from build123d import *

# Parameters (mm, degrees)
BOSS_EXTRUDE1_DEPTH     = 5
SKETCH2_W               = 3.5
SKETCH2_H               = 12
SKETCH2_W_2             = 3
BOSS_EXTRUDE2_DEPTH     = 20
SKETCH3_W               = 12
SKETCH3_H               = 3
SKETCH3_H_2             = 3.5
BOSS_EXTRUDE3_DEPTH     = 20
SKETCH4_W               = 5
SKETCH4_H               = 8
BOSS_EXTRUDE4_DEPTH     = 18
SKETCH5_R               = 3.5
CUT_EXTRUDE1_DEPTH      = 3.5
SKETCH6_R               = 3.5
CUT_EXTRUDE2_DEPTH      = 3.5
SKETCH7_R               = 1.625
CUT_EXTRUDE3_DEPTH      = 5
SKETCH8_R               = 2.5
CUT_EXTRUDE4_DEPTH      = 3
SKETCH9_R               = 2.5
CUT_EXTRUDE5_DEPTH      = 3
FILLET1_R               = 6
FILLET2_R               = 2
FILLET4_R               = 4
SURFACECUT2_START       = -20
SURFACECUT2_DEPTH       = 25
SURFACECUT2_START_2     = 5
SURFACECUT2_2_OUTLINE_W = 12
SURFACECUT2_2_OUTLINE_H = 3
SURFACECUT2_2_DEPTH     = 20


# Read off the part's stored shape, not the designer's step: SurfaceCut2
with BuildPart() as part:
    # Sketch1 → Boss-Extrude1 (new body)
    with BuildSketch(Plane.XY):
        Polygon((21.1, 0), (38.5, 0), (38.5, 12), (17.6, 12), (17.6, 26), (12.6, 26), (12.6, 12), (0, 12), (0, 0), (9.1, 0), (9.1, -26.5), (21.1, -26.5), align=None)
    extrude(amount=BOSS_EXTRUDE1_DEPTH)

    # Sketch2 → Boss-Extrude2 (add)
    with BuildSketch(Plane(origin=(0, 0, 0), x_dir=(-1, 0, 0), z_dir=(0, 0, -1))):
        with Locations((-1.75, 6)):
            Rectangle(SKETCH2_W, SKETCH2_H)
        with Locations((-37, 6)):
            Rectangle(SKETCH2_W_2, SKETCH2_H)
    extrude(amount=BOSS_EXTRUDE2_DEPTH)

    # Sketch3 → Boss-Extrude3 (add)
    with BuildSketch(Plane.XY.offset(5)):
        with Locations((15.1, -25)):
            Rectangle(SKETCH3_W, SKETCH3_H)
        with Locations((15.1, 10.25)):
            Rectangle(SKETCH3_W, SKETCH3_H_2)
    extrude(amount=BOSS_EXTRUDE3_DEPTH)

    # Sketch4 → Boss-Extrude4 (add)
    with BuildSketch(Plane(origin=(0, 0, 0), x_dir=(-1, 0, 0), z_dir=(0, 0, -1))):
        with Locations((-15.1, 22)):
            Rectangle(SKETCH4_W, SKETCH4_H)
    extrude(amount=BOSS_EXTRUDE4_DEPTH)

    # Sketch5 → Cut-Extrude1 (cut)
    with BuildSketch(Plane.ZY):
        with Locations((-14, 6)):
            Circle(SKETCH5_R)
    extrude(amount=-CUT_EXTRUDE1_DEPTH, mode=Mode.SUBTRACT)

    # Sketch6 → Cut-Extrude2 (cut)
    with BuildSketch(Plane(origin=(0, 12, 0), x_dir=(1, 0, 0), z_dir=(0, 1, 0))):
        with Locations(Location((15.1, -19, 0), (0, 0, 270))):
            Circle(SKETCH6_R)
    extrude(amount=-CUT_EXTRUDE2_DEPTH, mode=Mode.SUBTRACT)

    # Sketch7 → Cut-Extrude3 (cut)
    with BuildSketch(Plane.ZY.offset(-12.6)):
        with Locations((-14, 22)):
            Circle(SKETCH7_R)
    extrude(amount=-CUT_EXTRUDE3_DEPTH, mode=Mode.SUBTRACT)

    # Sketch8 → Cut-Extrude4 (cut)
    with BuildSketch(Plane.ZY.offset(-35.5)):
        with Locations((-14, 6)):
            Circle(SKETCH8_R)
    extrude(amount=-CUT_EXTRUDE4_DEPTH, mode=Mode.SUBTRACT)

    # Sketch9 → Cut-Extrude5 (cut)
    with BuildSketch(Plane(origin=(0, -23.5, 0), x_dir=(1, 0, 0), z_dir=(0, 1, 0))):
        with Locations(Location((15.1, -19, 0), (0, 0, 270))):
            Circle(SKETCH9_R)
    extrude(amount=-CUT_EXTRUDE5_DEPTH, mode=Mode.SUBTRACT)

    # Fillet1
    fillet1_edges = [part.edges().sort_by_distance(p)[0] for p in [
        (21.1, -25, 25),
        (9.1, -25, 25),
        (37, 0, -20),
        (37, 12, -20),
        (21.1, 10.25, 25),
        (9.1, 10.25, 25),
        (1.75, 0, -20),
        (1.75, 12, -20),
    ]]
    fillet(fillet1_edges, radius=FILLET1_R - 0.0001)  # a hair under: the kernel refuses the full size

    # Fillet2
    fillet2_edges = [part.edges().sort_by_distance(p)[0] for p in [
        (15.1, -26.5, 0),
        (38.5, 6, 5),
        (0, 6, 5),
        (15.1, 18, 0),
    ]]
    fillet(fillet2_edges, radius=FILLET2_R)

    # Fillet4
    fillet4_edges = [part.edges().sort_by_distance(p)[0] for p in [
        (15.1, 26, 5),
        (15.1, 26, -18),
        (15.1, 18, -18),
    ]]
    fillet(fillet4_edges, radius=FILLET4_R - 0.0001)  # a hair under: the kernel refuses the full size

    # SurfaceCut2 outline → SurfaceCut2 (cut)
    with BuildSketch(Plane.XY.offset(SURFACECUT2_START)):
        Polygon((0, 12), (0, 0), (9.1, 0), (9.1, -26.5), (21.1, -26.5), (21.1, 0), (38.5, 0), (38.5, 12), (17.6, 12), (17.6, 26), (12.6, 26), (12.6, 12), align=None)
    extrude(amount=SURFACECUT2_DEPTH, mode=Mode.SUBTRACT)

    # SurfaceCut2 2 outline → SurfaceCut2 2 (cut)
    with BuildSketch(Plane.XY.offset(SURFACECUT2_START_2)):
        with Locations((15.1, -25)):
            Rectangle(SURFACECUT2_2_OUTLINE_W, SURFACECUT2_2_OUTLINE_H)
    extrude(amount=SURFACECUT2_2_DEPTH, mode=Mode.SUBTRACT)


solid = part.part
Build history of the part. All positions in model axes, mm. Give positions to 0.01 mm unless a question says otherwise; leave off trailing zeros. Order: outer loops, then holes, each group sorted by start corner. A loop starts at its lowest first (then second) coordinate and runs counter-clockwise, first axis right, second up. Notation, with made-up numbers: M 49,6 L 54,6 A9 ccw 54,10 Z; hole C 79,-20.5 d4. An arc over 180 degrees is marked long. Put each result on its own line as item: value.
Item 1: Slice it at B-B, the plane x = 17.5. Write the cut outline in (y, z), plus the area to 3 significant figures.
From the geometry:
outline: M 8.5,5 L 12,5 L 12,16.45 L 8.5,16.45 Z; M 8.5,21.55 L 12,21.55 L 12,24.5 L 8.5,24.5 Z
area: 50.4 mm2
Item 2: Two-plate mould, pull along Z, no slides. Class faces 1 (the cylindrical face through (18.05, 10.27, 20.88)), 2 (the flat face through (15, 12, 13)), 3 (the flat face through (15, 10, 5)): +Z half, -Z half, draft (parallel to the pull), parting line (faces both ways), or undercut.
From the geometry:
face 1: undercut
face 2: draft
face 3: -Z half
Item 3: Probe line 1 (X direction, y = 10.4, z = 19); line 2 (Z direction, x = 12.5, y = 11.55); line 3 (Z direction, x = 13.5, y = 11.25). List the from-to ranges inside material, lowest first. Write a range as [from, to].
From the geometry:
line 1: x = [9.1, 11.6], [18.6, 21.1]
line 2: z = [5, 16.66], [21.34, 24.41]
line 3: z = [5, 15.89], [22.11, 24.78]
Item 4: Slice it at C-C, the plane z = 18.5. Write the cut outline in (x, y), plus the area to 3 significant figures.
From the geometry:
outline: M 9.1,8.5 L 11.64,8.5 L 11.64,12 L 9.1,12 Z; M 18.56,8.5 L 21.1,8.5 L 21.1,12 L 18.56,12 Z
area: 17.8 mm2
